The figure shows three views and two pictorial views of one solid part (mm, origin at its lowest corner). Answer the questions. Give positions to 0.01 mm unless a question says otherwise; leave off trailing zeros. Write each loop counter-clockwise with the first axis right and the second up, starting at its lowest first coordinate (ties: lowest second). Pieces come first, ordered by that corner, then holes. Notation, with made-up numbers: (-9.75, -23.75) - (38.25, -23.75) arc R17 ccw to (38.25, -6.75) - close; hole circle Ø8 at (39, 21.25). An arc over 180 degrees is marked (long way). Write each question's results on one line, items separated by ' | '. Start each with the question number.
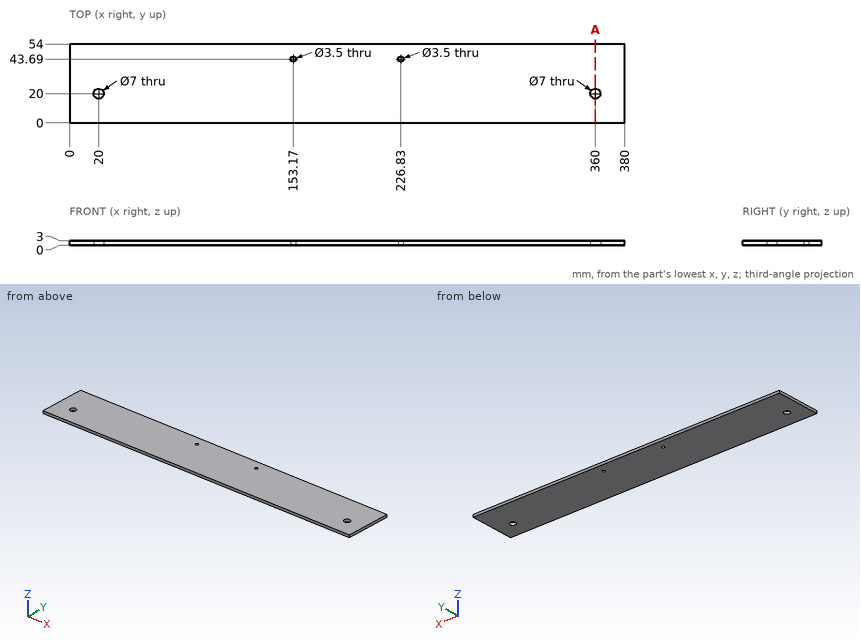
Q1. Consider L1, parallel to X at y = 43.69, z = 0.65; L2, parallel to Y at x = 153.17, z = 1.95; L3, parallel to Y at x = 20, z = 1.7. Determine where each line is inside the solid, lowest interval first.
Q2. Given pin 1 (6.5 mm diameter, centred on x = 20, y = 20, fed in from +Z); pin 2 (4 mm diameter, centred on x = 120, y = 16.5, fed in from -Z), each flat-ended and moving along its own axis, determine where each tip first touches the part or whether it passes through.
Q3. A cutting plane is placed at A-A, the plane x = 360. Write down the section's boundary in (y, z), and give its area (3 significant figures).
Result:
1) L1: x = 0 to 151.42, 154.92 to 225.08, 228.58 to 380 | L2: y = 0 to 41.94, 45.44 to 54 | L3: y = 0 to 16.5, 23.5 to 54
2) pin 1: passes through | pin 2: stops at z = 0
3) outline: (0, 0) - (16.5, 0) - (16.5, 3) - (0, 3) - close; (23.5, 0) - (54, 0) - (54, 3) - (23.5, 3) - close | area: 141 mm2
